from build123d import *

# Parameters (mm, degrees)
SKETCH_R             = 2.5
PAD_DEPTH            = 10
SKETCH001_R          = 12.5
PAD001_DEPTH         = 25
SKETCH002_R          = 7.5
POCKET_DEPTH         = 10
SKETCH003_W          = 5
SKETCH003_H          = 3.523945
POCKET001_DEPTH      = 5
POLARPATTERN_COUNT   = 2
PAD002_DEPTH         = 1.5
SKETCH005_R          = 3
POCKET002_DEPTH      = 28.248449
POCKET002_DEPTH_BACK = -3.753551
SKETCH006_W          = 15
SKETCH006_H          = 3
POCKET003_DEPTH      = 32.001


with BuildPart() as part:
    # Sketch → Pad (new body)
    with BuildSketch(Plane.XY):
        with BuildLine():
            ThreePointArc((-25, 16), (-29.242641, 14.242641), (-31, 10))
            Line((-31, -10), (-31, 10))
            ThreePointArc((-31, -10), (-29.242641, -14.242641), (-25, -16))
            Line((25, -16), (-25, -16))
            ThreePointArc((25, -16), (29.242641, -14.242641), (31, -10))
            Line((31, 10), (31, -10))
            ThreePointArc((31, 10), (29.242641, 14.242641), (25, 16))
            Line((-25, 16), (25, 16))
        make_face()
        with Locations((-25, -10)):
            Circle(SKETCH_R, mode=Mode.SUBTRACT)
        with Locations((-25, 10)):
            Circle(SKETCH_R, mode=Mode.SUBTRACT)
        with Locations((25, -10)):
            Circle(SKETCH_R, mode=Mode.SUBTRACT)
        with Locations((25, 10)):
            Circle(SKETCH_R, mode=Mode.SUBTRACT)
    extrude(amount=PAD_DEPTH)

    # Sketch001 (on Face14 of Pad) → Pad001 (join)
    with BuildSketch(Plane.XY.offset(10)):
        Circle(SKETCH001_R)
    extrude(amount=PAD001_DEPTH)

    # Sketch002 (on Face16 of Pad001) → Pocket (cut)
    with BuildSketch(Plane.XY.offset(35)):
        Circle(SKETCH002_R)
    extrude(amount=-POCKET_DEPTH, mode=Mode.SUBTRACT)

    # Sketch003 (on Face16 of Pocket) → Pocket001 (cut)
    with BuildSketch(Plane.XY.offset(35)):
        with Locations((0, 12.261972)):
            Rectangle(SKETCH003_W, SKETCH003_H)
    pocket001 = extrude(amount=-POCKET001_DEPTH, mode=Mode.SUBTRACT)

    # PolarPattern: Pocket001 ×2 about axis
    polarpattern_axis = Axis((0, 0, 35), (0, 0, 1))
    for i in range(1, POLARPATTERN_COUNT):
        add(pocket001.rotate(polarpattern_axis, i * 360 / POLARPATTERN_COUNT), mode=Mode.SUBTRACT)

    # Sketch004 (on DatumPlane) → Pad002 (join, symmetric)
    with BuildSketch(Plane(origin=(12.5, 0, 35), x_dir=(1, 0, 0), z_dir=(0, -1, 0))):
        Polygon((-0.2, -6), (3, -6), (12.5, -25), (-0.2, -25), align=None)
    pad002 = extrude(amount=PAD002_DEPTH, both=True)

    # Mirrored: Pad002 across YZ
    add(pad002.mirror(Plane.YZ))

    # Sketch005 (on DatumPlane) → Pocket002 (cut, two sides)
    with BuildSketch(Plane(origin=(0, -12.247449, 30), x_dir=(1, 0, 0), z_dir=(0, -1, 0))) as pocket002_sk:
        with Locations((0, -9)):
            Circle(SKETCH005_R)
    extrude(amount=-POCKET002_DEPTH, mode=Mode.SUBTRACT)
    extrude(pocket002_sk.sketch, amount=-POCKET002_DEPTH_BACK, mode=Mode.SUBTRACT)

    # Sketch006 (on Face8 of Pocket002) → Pocket003 (cut, through all)
    with BuildSketch(Plane.XZ.offset(16)):
        Rectangle(SKETCH006_W, SKETCH006_H)
    extrude(amount=-POCKET003_DEPTH, mode=Mode.SUBTRACT)


solid = part.part
The model under review builds one solid part; all positions refer to its coordinate system, in mm. A direction names the side the tool comes from. Give positions to 0.01 mm unless a question says otherwise; leave off trailing zeros. Write each loop counter-clockwise with the first axis right and the second up, starting at its lowest first coordinate (ties: lowest second). Pieces come first, ordered by that corner, then holes.
1. Add section C-C, the plane z = 14.5. Write out the cut boundary in (x, y).
2. Draft analysis for pull direction Y (two halves, no side actions). For faces 6 (the flat face through (-7, 11, 10)), 7 (the cylindrical face through (11.547, -4.788, 22.325)), 8 (the cylindrical face through (-27, 8.5, 4.9)), state which applies: +Y half, -Y half, draft (parallel to the pull), parting line (faces both ways), or undercut.
3. Add section D-D, the plane y = 0. Write out the cut boundary in (x, z), plus the area to 3 significant figures.
4. Add section B-B, the plane z = 32.5. Write out the cut boundary in (x, y), plus the area to 3 significant figures.
5. Add section A-A, the plane y = 8.5. Write out the cut boundary in (x, z).
6. Wall thickness on L1, parallel to Y at x = -25, z = 7.75; L2, parallel to Y at x = 0, z = 32.75; L3, parallel to X at y = -8.5, z = 2: over which ranges is each line inside the solid? List them lowest first.
7. For P1, Ø0.5, axis at y = -11.5, z = 32.5, coming from the -X side; P2, Ø2, axis at x = 10.5, z = 13.5, coming from the -Y side; P3, Ø0.5, axis at y = -11, z = 31.5, coming from the +X side, all flat-tipped, find the tip position at first contact; note any pin that passes through.
8. Tool access review of faces 1 (the flat face through (-17, -1.5, 18)), 2 (the flat face through (0, 10.5, 33)), 3 (the flat face through (2.5, -11, 33)), 4 (the flat face through (0, 16, 5)), 5 (the cylindrical face through (-7.493, 0.33, 30.07)): name each direction out of +Z, -Z, +X, -X, +Y, -Y from which nothing blocks a thin tool from reaching the whole face with its end or side.
Worked answers:
1. outline: (-22.75, -1.5) - (-12.41, -1.5) arc R12.5 ccw to (12.41, -1.5) - (22.75, -1.5) - (22.75, 1.5) - (12.41, 1.5) arc R12.5 ccw to (-12.41, 1.5) - (-22.75, 1.5) - close
2. face 6: draft
2. face 7: parting line
2. face 8: undercut
3. outline: (-31, 0) - (-7.5, 0) - (-7.5, 1.5) - (7.5, 1.5) - (7.5, 0) - (31, 0) - (31, 10) - (25, 10) - (15.5, 29) - (12.5, 29) - (12.5, 35) - (7.5, 35) - (7.5, 25) - (-7.5, 25) - (-7.5, 35) - (-12.5, 35) - (-12.5, 29) - (-15.5, 29) - (-25, 10) - (-31, 10) - close; hole circle Ø6 at (0, 21)
3. area: 1,340 mm2
4. outline: (-2.5, -12.25) - (-2.5, -10.5) - (2.5, -10.5) - (2.5, -12.25) arc R12.5 ccw to (2.5, 12.25) - (2.5, 10.5) - (-2.5, 10.5) - (-2.5, 12.25) arc R12.5 ccw to start; hole circle Ø15 at (0, 0)
4. area: 295 mm2
5. outline: (-31, 0) - (-27, 0) - (-27, 10) - (-31, 10) - close; (-23, 0) - (-7.5, 0) - (-7.5, 1.5) - (7.5, 1.5) - (7.5, 0) - (23, 0) - (23, 10) - (9.17, 10) - (9.17, 35) - (-9.17, 35) - (-9.17, 10) - (-23, 10) - close; (27, 0) - (31, 0) - (31, 10) - (27, 10) - close; hole circle Ø6 at (0, 21)
6. L1: y = -16 to -12.5, -7.5 to 7.5, 12.5 to 16
6. L2: y = -10.5 to -7.5, 7.5 to 10.5
6. L3: x = -31 to -27, -23 to 23, 27 to 31
7. P1: stops at x = -5.45
7. P2: stops at y = -8.12
7. P3: stops at x = 6.38
8. face 1: +Z, -X, -Y
8. face 2: +Z, +Y
8. face 3: +Z, -Y
8. face 4: +Z, -Z, +X, -X, +Y
8. face 5: +Z
